from build123d import *

# Parameters (mm, degrees)
SKETCH_R          = 51
SKETCH_R_2        = 34
PAD_DEPTH         = 1.5
SKETCH001_R       = 45
SKETCH001_R_2     = 42.5
PAD001_DEPTH      = 5
SKETCH002_R       = 43
SKETCH002_R_2     = 34
PAD002_DEPTH      = 2
SKETCH004_R       = 5
POCKET001_DEPTH   = 3.5
PAD003_DEPTH      = 3
SKETCH003_R       = 1.5
POCKET_DEPTH      = 3.501
POCKET_DEPTH_BACK = -3.001
CHAMFER_SIZE      = 1


with BuildPart() as part:
    # Sketch → Pad (new body)
    with BuildSketch(Plane.XY):
        Circle(SKETCH_R)
        Circle(SKETCH_R_2, mode=Mode.SUBTRACT)
    extrude(amount=PAD_DEPTH)

    # Sketch001 (on Face4 of Pad) → Pad001 (join)
    with BuildSketch(Plane.XY.offset(1.5)):
        Circle(SKETCH001_R)
        Circle(SKETCH001_R_2, mode=Mode.SUBTRACT)
    extrude(amount=PAD001_DEPTH)

    # Sketch002 (on Face6 of Pad001) → Pad002 (join)
    with BuildSketch(Plane.XY.offset(1.5)):
        Circle(SKETCH002_R)
        Circle(SKETCH002_R_2, mode=Mode.SUBTRACT)
    extrude(amount=PAD002_DEPTH)

    # Sketch004 → Pocket001 (cut)
    with BuildSketch(Plane(origin=(0, 0, 0), x_dir=(1, 0, 0), z_dir=(0, 0, -1))):
        with Locations((32.04294, 18.5)):
            Circle(SKETCH004_R)
        with Locations((-32.04294, 18.5)):
            Circle(SKETCH004_R)
        with Locations((0, -37)):
            Circle(SKETCH004_R)
    extrude(amount=-POCKET001_DEPTH, mode=Mode.SUBTRACT)

    # Sketch005 (on Face19 of Pocket001) → Pad003 (join)
    with BuildSketch(Plane.XY.offset(3.5)):
        with BuildLine():
            ThreePointArc((13.890561, 31.033084), (0.148301, 33.999677), (-13.619315, 31.153078))
            Line((-7.268789, 41.873795), (-13.619315, 31.153078))
            ThreePointArc((7.554436, 41.823205), (0.145046, 42.499752), (-7.268789, 41.873795))
            Line((13.890561, 31.033084), (7.554436, 41.823205))
        make_face()
        with BuildLine():
            ThreePointArc((-40.215676, -13.745888), (-36.969341, -20.96468), (-32.440728, -27.456314))
            Line((-32.440728, -27.456314), (-20.053698, -27.456314))
            ThreePointArc((-33.865149, -3.025171), (-29.597816, -16.732283), (-20.053698, -27.456314))
            Line((-33.865149, -3.025171), (-40.215676, -13.745888))
        make_face()
        with BuildLine():
            Line((40.204551, -13.778393), (33.868425, -2.988272))
            ThreePointArc((20.053698, -27.456314), (29.606927, -16.716156), (33.868425, -2.988272))
            Line((20.053698, -27.456314), (32.440728, -27.456314))
            ThreePointArc((32.440728, -27.456314), (36.960864, -20.979621), (40.204551, -13.778393))
        make_face()
    extrude(amount=PAD003_DEPTH)

    # Sketch003 (on Face8 of Pad002) → Pocket (cut, two sides)
    with BuildSketch(Plane.XY.offset(3.5)) as pocket_sk:
        with Locations((0, 37)):
            Circle(SKETCH003_R)
        with Locations((32.04294, -18.5)):
            Circle(SKETCH003_R)
        with Locations((-32.04294, -18.5)):
            Circle(SKETCH003_R)
    extrude(amount=-POCKET_DEPTH, mode=Mode.SUBTRACT)
    extrude(pocket_sk.sketch, amount=-POCKET_DEPTH_BACK, mode=Mode.SUBTRACT)

    # Chamfer
    chamfer_edges = [part.edges().sort_by_distance(p)[0] for p in [
        (-45, 0, 6.5),
    ]]
    chamfer(chamfer_edges, length=CHAMFER_SIZE)


solid = part.part
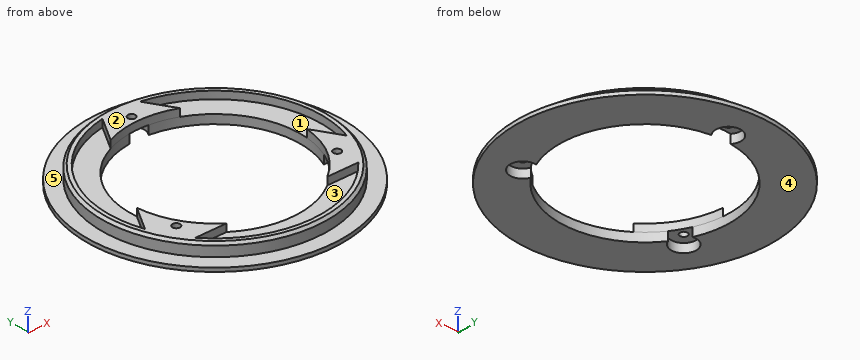
Geometry check sheet. Reference: the model listing, model coordinates, mm. Face numbers are marked on the shaded views. A direction names the side the tool comes from. Round coordinates to 2 decimals unless told otherwise and drop trailing zeros. Write each loop counter-clockwise with the first axis right and the second up, starting at its lowest first coordinate (ties: lowest second). Pieces come first, ordered by that corner, then holes. Notation, with made-up numbers: (-35, 42.5) - (-17, 42.5) arc R13 ccw to (-17, 57.5) - close; hole circle Ø9 at (-33.5, 87). An arc over 180 degrees is marked (long way). One line per item, written item: value.
1. Mould release check, pull along X, two halves, no side actions. Record for the marked faces 1, 2 and 3: released by +X, released by -X, zero draft, split by the parting line, or undercut.
The answers:
face 1: undercut
face 2: zero draft
face 3: undercut
2. Cross-section at A-A on x = 0. Record the boundary of the cut face in (y, z).
The answers:
outline: (-51, 0) - (-34, 0) - (-34, 3.5) - (-42.5, 3.5) - (-42.5, 6.5) - (-44, 6.5) - (-45, 5.5) - (-45, 1.5) - (-51, 1.5) - close; (34, 3.5) - (35.5, 3.5) - (35.5, 6.5) - (34, 6.5) - close; (38.5, 3.5) - (42, 3.5) - (42, 0) - (51, 0) - (51, 1.5) - (45, 1.5) - (45, 5.5) - (44, 6.5) - (38.5, 6.5) - close
3. Cross-section at C-C on y = -18.5. Give the number of separate pieces and of enclosed holes in the cut face, and give its area (3 significant figures).
The answers:
separate pieces: 4
enclosed holes: 0
area: 103 mm^2
4. Set-up check for the marked faces 4 and 5: record each of +Z, -Z, +X, -X, +Y, -Y from which the full face is reachable in a straight line by a thin tool's end or side.
The answers:
face 4: -Z, +X, -X, +Y, -Y
face 5: +Z
5. Cross-section at B-B on y = 0. Record the boundary of the cut face in (x, z), and give its area (3 significant figures).
The answers:
outline: (-51, 0) - (-34, 0) - (-34, 3.5) - (-42.5, 3.5) - (-42.5, 6.5) - (-44, 6.5) - (-45, 5.5) - (-45, 1.5) - (-51, 1.5) - close; (34, 0) - (51, 0) - (51, 1.5) - (45, 1.5) - (45, 5.5) - (44, 6.5) - (42.5, 6.5) - (42.5, 3.5) - (34, 3.5) - close
area: 109 mm^2
6. Depth check by flat-ended pin: pin 1 Ø2.5 at (x, z) = (-25.5, 5) entering from -Y; pin 2 Ø3 at (x, y) = (-34.5, 16) entering from +Z; pin 3 Ø4 at (x, y) = (32.04, -18.5) entering from +Z; pin 4 Ø3 at (x, z) = (28, 2) entering from -Y. Enter the tip coordinate at first touch or a pass-through.
The answers:
pin 1: stops at y = -37.91
pin 2: stops at z = 3.5
pin 3: stops at z = 6.5
pin 4: stops at y = -43.52
7. Scan lines: L1, parallel to Y at x = 9, z = 5.25; L2, parallel to Y at x = 31.5, z = 4.25; L3, parallel to X at y = 37, z = 5.5. Record each from-to range of solid material in increasing order.
The answers:
L1: y = -44.09 to -41.54, 32.79 to 39.36, 41.54 to 44.09
L2: y = -32.14 to -28.53, -27.46 to -19.9, -17.1 to -12.8, 28.53 to 32.14
L3: x = -25.61 to -20.91, -10.16 to -1.5, 1.5 to 10.39, 20.91 to 25.61
